```python
from build123d import *

# Parameters (mm, degrees)
SKETCH1_R                = 1
BOSS_EXTRUDE1_DEPTH      = 2
BOSS_EXTRUDE2_DEPTH      = 2
BOSS_EXTRUDE2_DEPTH_BACK = 2
FILLET1_R                = 2


with BuildPart() as part:
    # Sketch1 → Boss-Extrude1 (new body)
    with BuildSketch(Plane.XY):
        Polygon((-16, -14), (-16, 16), (14, 16), (14, -4), (4, -4), (4, -14), align=None)
        Circle(SKETCH1_R, mode=Mode.SUBTRACT)
    extrude(amount=BOSS_EXTRUDE1_DEPTH)

    # Sketch3 → Boss-Extrude2 (add, two sides: drawn at the far end of the back side and taken through both)
    with BuildSketch(Plane.XY.offset(2).offset(-BOSS_EXTRUDE2_DEPTH_BACK)):
        Polygon((-18, -14), (-16, -14), (-16, 16), (14, 16), (14, 18), (-18, 18), align=None)
    extrude(amount=BOSS_EXTRUDE2_DEPTH + BOSS_EXTRUDE2_DEPTH_BACK)

    # Fillet1
    fillet1_edges = [part.edges().sort_by_distance(p)[0] for p in [
        (14, 16, 3),
        (-16, -14, 3),
        (-18, 18, 2),
    ]]
    fillet(fillet1_edges, radius=FILLET1_R - 0.0001)  # a hair under: the kernel refuses the full size


solid = part.part
```
For this review, take the finished solid that the model builds, in its own axes (mm). A direction names the side the tool comes from. Give positions to 0.01 mm unless a question says otherwise; leave off trailing zeros. Order: outer loops, then holes, each group sorted by start corner. A loop starts at its lowest first (then second) coordinate and runs counter-clockwise, first axis right, second up.
1) Take a section at D-D (z = 0.65). Give the boundary of the cut face in (x, y).
2) The part is to be moulded in two halves that separate along X. For faces 1 (the face through (13.43, 16.6, 3.01)), 2 (the face through (-2, 16, 3)), 3 (the face through (0, -1, 1)), say which applies: released by +X, released by -X, zero draft, split by the parting line, or undercut.
3) Wall thickness on line 1 (Y direction, x = 0, z = 1.3); line 2 (X direction, y = 6.5, z = 2.9); line 3 (Y direction, x = 10.5, z = 1.7): over which ranges is each line inside the solid? List them lowest first.
4) Insertion check: pin 1 (12 mm diameter, centred on x = 4.5, y = 7.5, fed in from +Z); pin 2 (0.6 mm diameter, centred on y = -9, z = 0.5, fed in from +X); pin 3 (2 mm diameter, centred on x = 10, z = 1, fed in from -Y). Each pin has a flat end and moves straight along its axis. Give the tip position at first contact, or say it passes through.
5) Take a section at A-A (x = 0). Give the boundary of the cut face in (y, z).
6) For faces 4 (the face through (-2, 2, 2)), 5 (the face through (9, -4, 1)), 6 (the face through (-2, 2, 0)), list the 3-axis set-ups (+Z, -Z, +X, -X, +Y, -Y) from which the entire face can be reached by the end or side of a thin tool; tool diameter is ignored.
7) Take a section at B-B (y = 0). Give the boundary of the cut face in (x, z).
Derived:
1. outline: (-18, -14) - (4, -14) - (4, -4) - (14, -4) - (14, 18) - (-16, 18) arc R2 ccw to (-18, 16) - close; hole circle Ø2 at (0, 0)
2. face 1: released by +X
2. face 2: zero draft
2. face 3: undercut
3. line 1: y = -14 to -1, 1 to 18
3. line 2: x = -18 to -16
3. line 3: y = -4 to 18
4. pin 1: stops at z = 2
4. pin 2: stops at x = 4
4. pin 3: stops at y = -4
5. outline: (-14, 0) - (-1, 0) - (-1, 2) - (-14, 2) - close; (1, 0) - (18, 0) - (18, 4) - (16, 4) - (16, 2) - (1, 2) - close
6. face 4: +Z, +X, -Y
6. face 5: +Z, -Z, +X, -Y
6. face 6: -Z, +X, -X, +Y, -Y
7. outline: (-18, 0) - (-1, 0) - (-1, 2) - (-16, 2) - (-16, 4) - (-18, 4) - close; (1, 0) - (14, 0) - (14, 2) - (1, 2) - close
